Read the model definition and answer for the solid it produces. Units are mm, in the model's axes. Face numbers are marked on the shaded views. A direction names the side the tool comes from. Round coordinates to 2 decimals unless told otherwise and drop trailing zeros. Order: outer loops, then holes, each group sorted by start corner. A loop starts at its lowest first (then second) coordinate and runs counter-clockwise, first axis right, second up. Notation, with made-up numbers: (84.25, 62.5) - (124.25, 62.5) arc R29 ccw to (124.25, 90.5) - close; hole circle Ø7 at (12.25, 87). An arc over 180 degrees is marked (long way). Answer as a JSON object with one key per item and string values. Group by question number.
Q1. A tool of negligible diameter and unlimited length cuts with its end or side. For the marked faces 4 and 5, from which of +Z, -Z, +X, -X, +Y, -Y can it reach the whole face along a straight path? Write none if from no direction.
Q2. The mould has two halves that part along Z. Classify the marked faces 1, 2 and 3: pulls with the +Z half, pulls with the -Z half, needs draft (parallel to the pull), parting line crosses it, or undercut.
Q3. Given pin 1 Ø2 at (x, z) = (-6.5, 11.5) entering from -Y (3 decimals); pin 2 Ø2 at (x, z) = (7, 11) entering from +Y; pin 3 Ø2 at (y, z) = (7, 11) entering from +X; pin 4 Ø2.5 at (x, y) = (0, 0) entering from -Z, each flat-ended and moving along its own axis, determine where each tip first touches the part or whether it passes through.
Q4. Consider line 1 (Y direction, x = 0, z = 7) (3 decimals); line 2 (Y direction, x = 0.75, z = 5.25); line 3 (X direction, y = 0.25, z = 6). Determine where each line is inside the solid, lowest interval first.
Q5. A cutting plane is placed at B-B on z = 11.5. Determine the outline of the cut face in (x, y) (3 decimals).
Q6. A cutting plane is placed at A-A on z = 5.75. Determine the outline of the cut face in (x, y) (3 decimals).
Q7. A cutting plane is placed at C-C on y = -7. Count the separate pieces of the cut face and the enclosed holes in it, and give its area (3 significant figures).
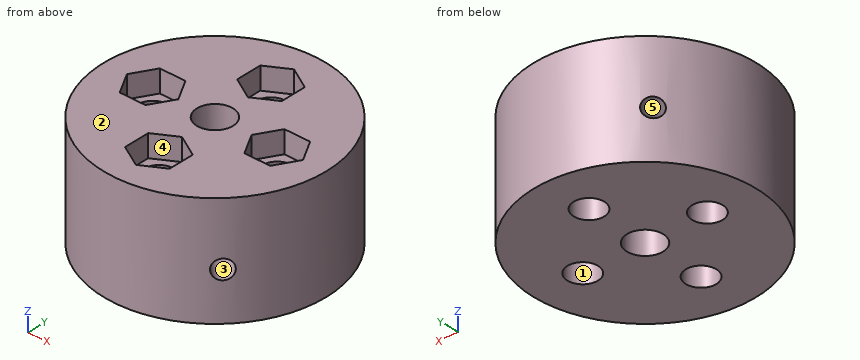
```python
from build123d import *

# Parameters (mm, degrees)
SKETCH1_R               = 12.5
BOSS_EXTRUDE1_DEPTH     = 12.5
SKETCH2_R               = 1.71
CUT_EXTRUDE1_DEPTH      = 2.5
CUT_EXTRUDE2_START      = -12.5
SKETCH2_3_R             = 1.71
CUT_EXTRUDE2_DEPTH      = 10
CIRPATTERN1_COUNT       = 4
CUT_EXTRUDE3_REACH      = 14.5
SKETCH3_R               = 2.025
SKETCH6_R               = 1.08
CUT_EXTRUDE5_DEPTH      = 18.67766953
CUT_EXTRUDE5_DEPTH_BACK = 18.67766953


with BuildPart() as part:
    # Sketch1 → Boss-Extrude1 (new body)
    with BuildSketch(Plane.XY):
        Circle(SKETCH1_R)
    extrude(amount=BOSS_EXTRUDE1_DEPTH)

    # Sketch2 → Cut-Extrude1 (cut)
    with BuildSketch(Plane.XY.offset(12.5)):
        Polygon((2.5, 5.556624327), (2.5, 8.443375673), (0, 9.886751346), (-2.5, 8.443375673), (-2.5, 5.556624327), (0, 4.113248654), align=None)
        with Locations((0, 7)):
            Circle(SKETCH2_R, mode=Mode.SUBTRACT)
        with Locations((0, 7)):
            Circle(SKETCH2_R)
    cut_extrude1 = extrude(amount=-CUT_EXTRUDE1_DEPTH, mode=Mode.SUBTRACT)

    # Sketch2_3 → Cut-Extrude2 (cut)
    with BuildSketch(Plane.XY.offset(12.5).offset(CUT_EXTRUDE2_START)):
        with Locations((0, 7)):
            Circle(SKETCH2_3_R)
    cut_extrude2 = extrude(amount=CUT_EXTRUDE2_DEPTH, mode=Mode.SUBTRACT)

    # CirPattern1: Cut-Extrude1, Cut-Extrude2 ×4 about axis
    cirpattern1_axis = Axis((0, 0, 0), (0, 0, 1))
    for i in range(1, CIRPATTERN1_COUNT):
        add(cut_extrude1.rotate(cirpattern1_axis, i * 360 / CIRPATTERN1_COUNT), mode=Mode.SUBTRACT)
        add(cut_extrude2.rotate(cirpattern1_axis, i * 360 / CIRPATTERN1_COUNT), mode=Mode.SUBTRACT)

    # Sketch3 → Cut-Extrude3 (cut, up to next)
    with BuildSketch(Plane.XY.offset(12.5), mode=Mode.PRIVATE) as cut_extrude3_sk1:
        Circle(SKETCH3_R)
    cut_extrude3_tool1 = extrude(cut_extrude3_sk1.sketch, amount=-CUT_EXTRUDE3_REACH, mode=Mode.PRIVATE) & part.part
    add(cut_extrude3_tool1.solids().sort_by_distance((0, 0, 12.5))[0], mode=Mode.SUBTRACT)

    # Sketch6 → Cut-Extrude5 (cut, two sides)
    with BuildSketch(Plane(origin=(0, 0, 0), x_dir=(0.707106781, 0.707106781, 0), z_dir=(-0.707106781, 0.707106781, 0))) as cut_extrude5_sk:
        with Locations((0, -5.41)):
            Circle(SKETCH6_R)
    extrude(amount=CUT_EXTRUDE5_DEPTH, mode=Mode.SUBTRACT)
    extrude(cut_extrude5_sk.sketch, amount=-CUT_EXTRUDE5_DEPTH_BACK, mode=Mode.SUBTRACT)


solid = part.part
```
Result set:
{
 "1": {"face 4": "+Z", "face 5": "none"},
 "2": {"face 1": "needs draft", "face 2": "pulls with the +Z half", "face 3": "undercut"},
 "3": {"pin 1": "stops at y = -11.225", "pin 2": "stops at y = 10.97", "pin 3": "stops at x = 10.97", "pin 4": "passes through"},
 "4": {"line 1": "y = -12.5 to -8.71, -5.29 to -2.025, 2.025 to 5.29, 8.71 to 12.5", "line 2": "y = -12.48 to -8.54, -5.46 to -2.26, 1.88 to 5.46, 8.54 to 12.48", "line 3": "x = -12.5 to -8.69, -5.31 to -2.01, 2.01 to 5.31, 8.69 to 12.5"},
 "5": {"outline": "circle Ø25 at (0, 0); hole (-9.887, 0) - (-8.443, -2.5) - (-5.557, -2.5) - (-4.113, 0) - (-5.557, 2.5) - (-8.443, 2.5) - close; hole (-2.5, -8.443) - (0, -9.887) - (2.5, -8.443) - (2.5, -5.557) - (0, -4.113) - (-2.5, -5.557) - close; hole (-2.5, 5.557) - (0, 4.113) - (2.5, 5.557) - (2.5, 8.443) - (0, 9.887) - (-2.5, 8.443) - close; hole circle Ø4.05 at (0, 0); hole (4.113, 0) - (5.557, -2.5) - (8.443, -2.5) - (9.887, 0) - (8.443, 2.5) - (5.557, 2.5) - close"},
 "6": {"outline": "(-9.534, 8.084) arc R12.5 ccw to (8.084, -9.534) - (0.51, -1.96) arc R2.025 cw to (-1.96, 0.51) - close; (-8.084, 9.534) - (-0.51, 1.96) arc R2.025 cw to (1.96, -0.51) - (9.534, -8.084) arc R12.5 ccw to start; hole circle Ø3.42 at (-7, 0); hole circle Ø3.42 at (0, -7); hole circle Ø3.42 at (0, 7); hole circle Ø3.42 at (7, 0)"},
 "7": {"separate pieces": "2", "enclosed holes": "1", "area": "207 mm²"}
}
